For this review, use the dimensioned drawing (mm, ordinates from the lowest corner) and the shaded views. A direction names the side the tool comes from. Coordinates: 2 decimals unless noted, no trailing zeros. Loops run counter-clockwise (first coordinate to the right, second up) from the corner with the lowest first, then second, coordinate; pieces in that order, holes last. Notation, with made-up numbers: (55, -30.75) -> (84, -30.75) arc R31 cw to (84, -5.75) -> close; hole circle Ø1 at (22.25, 40). An arc over 180 degrees is marked (long way). Use one line per item in the form item = value. Start each with the question number.
1. Consider section B-B (z = 9). State the section outline as (x, y) points.
2. Machinability: for the marked faces 1 and 2, which of the approach directions +Z, -Z, +X, -X, +Y, -Y give a long, thin tool a straight path to every point of the face, cutting with its end or side? Answer none if there is none.
3. Consider section D-D (x = 195.5). State the section outline as (y, z) points.
4. Consider section C-C (y = 9). State the section outline as (x, z) points.
5. For pin 1 (3 mm diameter, centred on x = 56.5, z = 15.5, fed in from +Y); pin 2 (12 mm diameter, centred on x = 206, z = 5.5, fed in from +Y); pin 3 (3 mm diameter, centred on x = 204, z = 23, fed in from -Y), all flat-tipped, find the tip position at first contact; note any pin that passes through.
6. Wall thickness on line 1 (Y direction, x = 73.5, z = 20.5); line 2 (X direction, y = 18, z = 37); line 3 (X direction, y = 6, z = 31.5): over which ranges is each line inside the solid? List them lowest first. Write a range as from..to.
7. Consider section A-A (x = 107.5). State the section outline as (y, z) points.
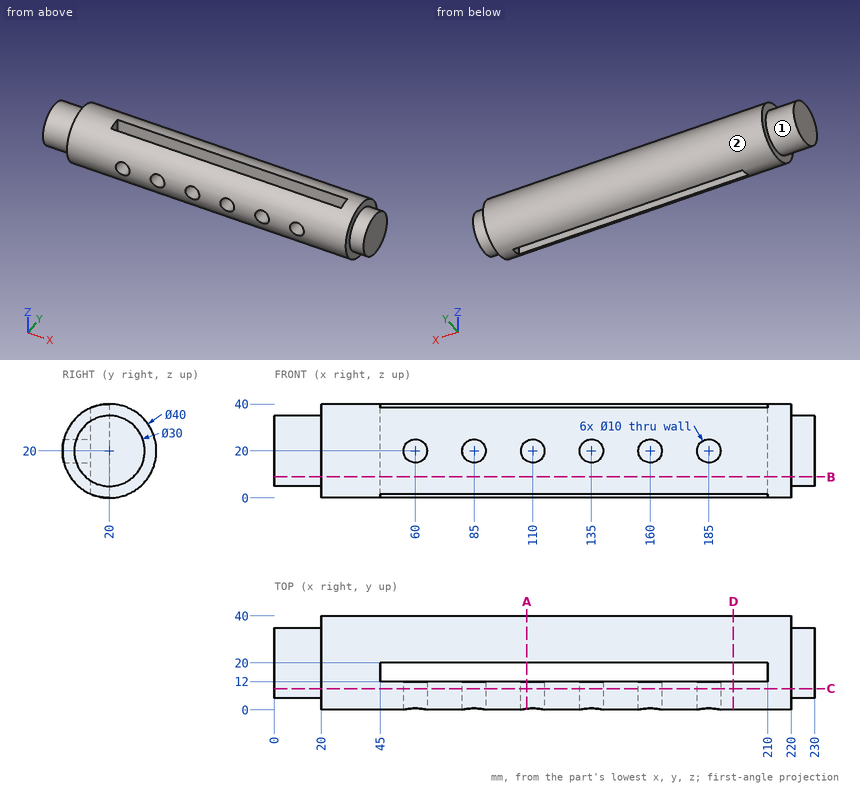
Geometry check:
q1.outline = (0, 9.8) -> (20, 9.8) -> (20, 3.3) -> (220, 3.3) -> (220, 9.8) -> (230, 9.8) -> (230, 30.2) -> (220, 30.2) -> (220, 36.7) -> (20, 36.7) -> (20, 30.2) -> (0, 30.2) -> close; hole (45, 12) -> (210, 12) -> (210, 20) -> (45, 20) -> close
q2.face_1 = -X
q2.face_2 = +X, -X
q3.outline = (12, 1.67) -> (12, 38.33) arc R20 ccw to start; (20, 0) arc R20 ccw to (20, 40) -> close
q4.outline = (0, 9.8) -> (20, 9.8) -> (20, 3.3) -> (220, 3.3) -> (220, 9.8) -> (230, 9.8) -> (230, 30.2) -> (220, 30.2) -> (220, 36.7) -> (20, 36.7) -> (20, 30.2) -> (0, 30.2) -> close; hole circle Ø10 at (60, 20); hole circle Ø10 at (85, 20); hole circle Ø10 at (110, 20); hole circle Ø10 at (135, 20); hole circle Ø10 at (160, 20); hole circle Ø10 at (185, 20)
q5.pin_1 = 39.77
q5.pin_2 = 38.1
q5.pin_3 = 0.06
q6.line_1 = 0.01..12, 20..39.99
q6.line_2 = 20..45, 210..220
q6.line_3 = 20..220
q7.outline = (0.47, 15.67) arc R20 ccw to (12, 1.67) -> (12, 15.67) -> close; (0.47, 24.33) -> (12, 24.33) -> (12, 38.33) arc R20 ccw to start; (20, 0) arc R20 ccw to (20, 40) -> close
